Could you check a few things on this model? Use its own coordinates, in mm. Face numbers are marked on the shaded views. Round coordinates to 2 decimals unless told otherwise and drop trailing zeros. Write each loop counter-clockwise with the first axis right and the second up, starting at its lowest first coordinate (ties: lowest second). Pieces come first, ordered by that corner, then holes. Notation, with made-up numbers: (58, -1) -> (69, -1) arc R22 ccw to (69, 14) -> close; hole circle Ø3 at (-22, 18.25). An arc over 180 degrees is marked (long way). Return JSON: item names as keys, results as strings.
from build123d import *

# Parameters (mm, degrees)
F0_R     = 12.7
F1_DEPTH = 127
F2_R     = 25.4
F3_DEPTH = 12.7
F5_R     = 6.35
F6_DEPTH = 38.101


with BuildPart() as f1:
    # F0 (on Right) → F1 (new body)
    with BuildSketch(Plane.YZ):
        Circle(F0_R)
    extrude(amount=F1_DEPTH)

    # F2 (on face) → F3 (join)
    with BuildSketch(Plane(origin=(0, 0, 0), x_dir=(0, -1, 0), z_dir=(-1, 0, 0))):
        Circle(F2_R)
    extrude(amount=F3_DEPTH)

    # F5 (on offset) → F6 (cut, through all)
    with BuildSketch(Plane.XY.offset(12.7)):
        with Locations((113.03, 0)):
            Circle(F5_R)
    extrude(amount=-F6_DEPTH, mode=Mode.SUBTRACT)


solid = f1.part
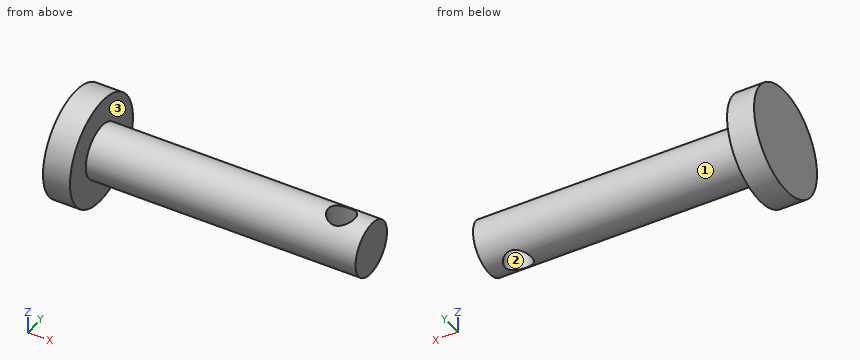
1) I want a section at A-A, the plane y = 0. Please give me the cut outline in (x, z), and give its area (3 significant figures).
Return value:
{"outline": "(-12.7, -25.4) -> (0, -25.4) -> (0, -12.7) -> (106.68, -12.7) -> (106.68, 12.7) -> (0, 12.7) -> (0, 25.4) -> (-12.7, 25.4) -> close; (119.38, -12.7) -> (127, -12.7) -> (127, 12.7) -> (119.38, 12.7) -> close", "area": "3,550 mm²"}
2) I want a section at B-B, the plane z = 0. Please give me the cut outline in (x, y).
Return value:
{"outline": "(-12.7, -25.4) -> (0, -25.4) -> (0, -12.7) -> (127, -12.7) -> (127, 12.7) -> (0, 12.7) -> (0, 25.4) -> (-12.7, 25.4) -> close; hole circle Ø12.7 at (113.03, 0)"}
3) If I drill on probe 1 along Y at (x, z) = (113.03, 0.5); probe 2 along X at (y, z) = (0, -4); probe 3 along Y at (x, z) = (60, -11), over which ranges is the centre line in solid material (lowest first)? Write a range as [from, to].
Return value:
{"probe 1": "[-12.69, -6.35], [6.35, 12.69]", "probe 2": "[-12.7, 106.68], [119.38, 127]", "probe 3": "[-6.35, 6.35]"}
4) Thinking about a two-plate mould opening in Y: for the marked faces 1, 2 and 3, which applies, pulls with the +Y half, pulls with the -Y half, needs draft (parallel to the pull), parting line crosses it, or undercut?
Return value:
{"face 1": "parting line crosses it", "face 2": "undercut", "face 3": "needs draft"}
5) I want a section at C-C, the plane x = 113.03. Please give me the cut outline in (y, z), and give its area (3 significant figures).
Return value:
{"outline": "(-6.35, -11) -> (-6.35, 11) arc R12.7 ccw to start; (6.35, -11) arc R12.7 ccw to (6.35, 11) -> close", "area": "198 mm²"}
6) Will these pins go through, and if not, where does the flat tip stop? pin 1 Ø8 at (x, z) = (70, 1.5) entering from +Y; pin 2 Ø8 at (x, z) = (63, 7) entering from +Y; pin 3 Ø6 at (x, y) = (31.5, 11) entering from -Z.
Return value:
{"pin 1": "y = 12.7", "pin 2": "y = 12.34", "pin 3": "z = -9.86"}
7) I want a section at D-D, the plane x = 70. Please give me the cut outline in (y, z), and give its area (3 significant figures).
Return value:
{"outline": "circle Ø25.4 at (0, 0)", "area": "507 mm²"}
